Design review of the part built by this model. Coordinates are the model's own, in mm. Face numbers are marked on the shaded views. A direction names the side the tool comes from. Coordinates: 2 decimals unless noted, no trailing zeros. Order: outer loops, then holes, each group sorted by start corner. A loop starts at its lowest first (then second) coordinate and runs counter-clockwise, first axis right, second up. Notation, with made-up numbers: (32.5, -6) -> (86.5, -6) arc R19 cw to (86.5, 25) -> close; hole circle Ø1 at (13, -5). An arc over 180 degrees is marked (long way). Write item = value, one per line.
```python
from build123d import *

# Parameters (mm, degrees)
SCHIZZO1_W                        = 69
SCHIZZO1_H                        = 49
ESTRUSIONE_ESTRUSIONE1_DEPTH      = 3
RACCORDO1_R                       = 1
RACCORDO2_R                       = 1
RACCORDO3_R                       = 1
RACCORDO4_R                       = 1
SCHIZZO2_W                        = 60
SCHIZZO2_H                        = 2.231214474
ESTRUSIONE_ESTRUSIONE2_DEPTH      = 3
RACCORDO5_R                       = 3
RACCORDO6_R                       = 3
SCHIZZO3_R                        = 1
TAGLIO_ESTRUSIONE1_DEPTH          = 3
SCHIZZO4_W                        = 24
SCHIZZO4_H                        = 14
TAGLIO_ESTRUSIONE2_DEPTH          = 3
SCHIZZO5_W                        = 23
SCHIZZO5_H                        = 23
TAGLIO_ESTRUSIONE3_DEPTH          = 1.2
RACCORDO7_R                       = 0.5
RACCORDO8_R                       = 0.5
RACCORDO9_R                       = 0.5
RACCORDO10_R                      = 0.5
RACCORDO11_R                      = 2
RACCORDO12_R                      = 2
RACCORDO13_R                      = 2
RACCORDO14_R                      = 2
SCHIZZO6_W                        = 8.444052449
SCHIZZO6_H                        = 8.25
ESTRUSIONE_ESTRUSIONE3_DEPTH      = 6
SCHIZZO7_R                        = 0.9
TAGLIO_ESTRUSIONE4_DEPTH          = 6
ESTRUSIONE_ESTRUSIONE4_DEPTH      = 1.2
ESTRUSIONE_ESTRUSIONE4_DEPTH_BACK = 3
SCHIZZO8_R                        = 1.75
TAGLIO_ESTRUSIONE5_DEPTH          = 3
TAGLIO_ESTRUSIONE6_DEPTH          = 2
SCHIZZO13_R                       = 1.9
ESTRUSIONE_ESTRUSIONE5_DEPTH      = 3.2
SCHIZZO14_R                       = 1.9
ESTRUSIONE_ESTRUSIONE6_DEPTH      = 3.2


with BuildPart() as part:
    # Schizzo1 → Estrusione-Estrusione1 (new body)
    with BuildSketch(Plane(origin=(0, 0, 0), x_dir=(1, 0, 0), z_dir=(0, 1, 0))):
        Rectangle(SCHIZZO1_W, SCHIZZO1_H)
    extrude(amount=ESTRUSIONE_ESTRUSIONE1_DEPTH)

    # Raccordo1
    raccordo1_edges = [part.edges().sort_by_distance(p)[0] for p in [
        (-34.5, 1.5, 24.5),
    ]]
    fillet(raccordo1_edges, radius=RACCORDO1_R)

    # Raccordo2
    raccordo2_edges = [part.edges().sort_by_distance(p)[0] for p in [
        (-34.5, 1.5, -24.5),
    ]]
    fillet(raccordo2_edges, radius=RACCORDO2_R)

    # Raccordo3
    raccordo3_edges = [part.edges().sort_by_distance(p)[0] for p in [
        (34.5, 1.5, 24.5),
    ]]
    fillet(raccordo3_edges, radius=RACCORDO3_R)

    # Raccordo4
    raccordo4_edges = [part.edges().sort_by_distance(p)[0] for p in [
        (34.5, 1.5, -24.5),
    ]]
    fillet(raccordo4_edges, radius=RACCORDO4_R)

    # Schizzo2 → Estrusione-Estrusione2 (add)
    with BuildSketch(Plane.XZ):
        with Locations((0, 21.334392763)):
            Rectangle(SCHIZZO2_W, SCHIZZO2_H)
        with Locations((0, -21.334392763)):
            Rectangle(SCHIZZO2_W, SCHIZZO2_H)
    extrude(amount=ESTRUSIONE_ESTRUSIONE2_DEPTH)

    # Raccordo5
    raccordo5_edges = [part.edges().sort_by_distance(p)[0] for p in [
        (0, 0, 20.218785526),
    ]]
    fillet(raccordo5_edges, radius=RACCORDO5_R - 0.0001)  # a hair under: the kernel refuses the full size

    # Raccordo6
    raccordo6_edges = [part.edges().sort_by_distance(p)[0] for p in [
        (0, 0, -20.218785526),
    ]]
    fillet(raccordo6_edges, radius=RACCORDO6_R - 0.0001)  # a hair under: the kernel refuses the full size

    # Schizzo3 → Taglio-Estrusione1 (cut)
    with BuildSketch(Plane(origin=(0, 3, 0), x_dir=(1, 0, 0), z_dir=(0, 1, 0))):
        with Locations(Location((-32.5, 22.5, 0), (0, 0, 270))):
            Circle(SCHIZZO3_R)
        with Locations(Location((32.5, 22.5, 0), (0, 0, 270))):
            Circle(SCHIZZO3_R)
        with Locations(Location((32.5, -22.5, 0), (0, 0, 270))):
            Circle(SCHIZZO3_R)
        with Locations(Location((-32.5, -22.5, 0), (0, 0, 270))):
            Circle(SCHIZZO3_R)
    extrude(amount=-TAGLIO_ESTRUSIONE1_DEPTH, mode=Mode.SUBTRACT)

    # Schizzo4 → Taglio-Estrusione2 (cut)
    with BuildSketch(Plane.XZ):
        with Locations((9.5, 0)):
            Rectangle(SCHIZZO4_W, SCHIZZO4_H)
    extrude(amount=-TAGLIO_ESTRUSIONE2_DEPTH, mode=Mode.SUBTRACT)

    # Schizzo5 → Taglio-Estrusione3 (cut)
    with BuildSketch(Plane.XZ):
        with Locations((-21.5, 0)):
            Rectangle(SCHIZZO5_W, SCHIZZO5_H)
    extrude(amount=-TAGLIO_ESTRUSIONE3_DEPTH, mode=Mode.SUBTRACT)

    # Raccordo7
    raccordo7_edges = [part.edges().sort_by_distance(p)[0] for p in [
        (-33, 0.6, 11.5),
    ]]
    fillet(raccordo7_edges, radius=RACCORDO7_R)

    # Raccordo8
    raccordo8_edges = [part.edges().sort_by_distance(p)[0] for p in [
        (-10, 0.6, 11.5),
    ]]
    fillet(raccordo8_edges, radius=RACCORDO8_R)

    # Raccordo9
    raccordo9_edges = [part.edges().sort_by_distance(p)[0] for p in [
        (-33, 0.6, -11.5),
    ]]
    fillet(raccordo9_edges, radius=RACCORDO9_R)

    # Raccordo10
    raccordo10_edges = [part.edges().sort_by_distance(p)[0] for p in [
        (-10, 0.6, -11.5),
    ]]
    fillet(raccordo10_edges, radius=RACCORDO10_R)

    # Raccordo11
    raccordo11_edges = [part.edges().sort_by_distance(p)[0] for p in [
        (21.5, 3, 0),
    ]]
    fillet(raccordo11_edges, radius=RACCORDO11_R)

    # Raccordo12
    raccordo12_edges = [part.edges().sort_by_distance(p)[0] for p in [
        (10.5, 3, 7),
    ]]
    fillet(raccordo12_edges, radius=RACCORDO12_R)

    # Raccordo13
    raccordo13_edges = [part.edges().sort_by_distance(p)[0] for p in [
        (-2.5, 3, 1),
    ]]
    fillet(raccordo13_edges, radius=RACCORDO13_R)

    # Raccordo14
    raccordo14_edges = [part.edges().sort_by_distance(p)[0] for p in [
        (9.5, 3, -7),
    ]]
    fillet(raccordo14_edges, radius=RACCORDO14_R)

    # Schizzo6 → Estrusione-Estrusione3 (add)
    with BuildSketch(Plane.XZ):
        with Locations((-6.722026225, 18.375)):
            Rectangle(SCHIZZO6_W, SCHIZZO6_H)
        with Locations((-6.722026225, -18.375)):
            Rectangle(SCHIZZO6_W, SCHIZZO6_H)
    extrude(amount=ESTRUSIONE_ESTRUSIONE3_DEPTH)

    # Schizzo7 → Taglio-Estrusione4 (cut)
    with BuildSketch(Plane.XZ.offset(6)):
        with Locations(Location((-6.72, 18.375, 0), (0, 0, 270))):
            Circle(SCHIZZO7_R)
        with Locations(Location((-6.72, -18.375, 0), (0, 0, 90))):
            Circle(SCHIZZO7_R)
    extrude(amount=-TAGLIO_ESTRUSIONE4_DEPTH, mode=Mode.SUBTRACT)

    # Schizzo8 → Estrusione-Estrusione4 (add, two sides: drawn at the far end of the back side and taken through both)
    with BuildSketch(Plane.XZ.offset(-ESTRUSIONE_ESTRUSIONE4_DEPTH_BACK)):
        with Locations(Location((28.5, 8.7, 0), (0, 0, 270))):
            Circle(SCHIZZO8_R)
        with Locations(Location((28.5, -8.7, 0), (0, 0, 90))):
            Circle(SCHIZZO8_R)
    extrude(amount=ESTRUSIONE_ESTRUSIONE4_DEPTH + ESTRUSIONE_ESTRUSIONE4_DEPTH_BACK)

    # Schizzo9 → Taglio-Estrusione5 (cut)
    with BuildSketch(Plane.XZ):
        with BuildLine():
            Line((28.523054823, 11.139507375), (23.522221501, 11.139507375))
            Line((23.522221501, 11.139507375), (23.522221501, 11.920576973))
            Line((23.522221501, 11.920576973), (28.476945177, 11.920576973))
            ThreePointArc((28.476945177, 11.920576973), (30.793594038, 10.980088836), (31.766686618, 8.676945177))
            ThreePointArc((31.766686618, 8.676945177), (30.793594038, 6.373801519), (28.476945177, 5.433313382))
            Line((28.476945177, 5.433313382), (23.522221501, 5.433313382))
            Line((23.522221501, 5.433313382), (23.522221501, 6.21438298))
            Line((23.522221501, 6.21438298), (28.523054823, 6.21438298))
            ThreePointArc((28.523054823, 6.21438298), (30.241294429, 6.945200369), (30.939507375, 8.676945177))
            ThreePointArc((30.939507375, 8.676945177), (30.241294429, 10.408689986), (28.523054823, 11.139507375))
        make_face()
        with BuildLine():
            Line((23.522221501, -5.433313382), (23.522221501, -6.21438298))
            Line((23.522221501, -6.21438298), (28.523054823, -6.21438298))
            ThreePointArc((28.523054823, -6.21438298), (30.241294429, -6.945200369), (30.939507375, -8.676945177))
            ThreePointArc((30.939507375, -8.676945177), (30.241294429, -10.408689986), (28.523054823, -11.139507375))
            Line((28.523054823, -11.139507375), (23.522221501, -11.139507375))
            Line((23.522221501, -11.139507375), (23.522221501, -11.920576973))
            Line((23.522221501, -11.920576973), (28.476945177, -11.920576973))
            ThreePointArc((28.476945177, -11.920576973), (30.793594038, -10.980088836), (31.766686618, -8.676945177))
            ThreePointArc((31.766686618, -8.676945177), (30.793594038, -6.373801519), (28.476945177, -5.433313382))
            Line((28.476945177, -5.433313382), (23.522221501, -5.433313382))
        make_face()
    extrude(amount=-TAGLIO_ESTRUSIONE5_DEPTH, mode=Mode.SUBTRACT)

    # Schizzo11 → Taglio-Estrusione6 (cut)
    with BuildSketch(Plane.XZ):
        with BuildLine():
            Line((28.523054823, 11.139507375), (23.522221501, 11.139507375))
            Line((23.522221501, 11.139507375), (23.522221501, 6.21438298))
            Line((23.522221501, 6.21438298), (28.523054823, 6.21438298))
            ThreePointArc((28.523054823, 6.21438298), (30.248124061, 6.938498616), (30.939507375, 8.676945177))
            ThreePointArc((30.939507375, 8.676945177), (30.248124061, 10.415391738), (28.523054823, 11.139507375))
        make_face()
        with BuildLine():
            Line((23.522221501, -6.21438298), (28.523054823, -6.21438298))
            ThreePointArc((28.523054823, -6.21438298), (30.248124061, -6.938498616), (30.939507375, -8.676945177))
            ThreePointArc((30.939507375, -8.676945177), (30.248124061, -10.415391738), (28.523054823, -11.139507375))
            Line((28.523054823, -11.139507375), (23.522221501, -11.139507375))
            Line((23.522221501, -11.139507375), (23.522221501, -6.21438298))
        make_face()
    extrude(amount=-TAGLIO_ESTRUSIONE6_DEPTH, mode=Mode.SUBTRACT)


with BuildPart() as taglio_estrusione6_piece_1:
    # of the separate pieces the step leaves, piece 1, a body of its own (taglio_estrusione6_pieces)
    add(part.part.solids().sort_by_distance((34.5, 3, -23.5))[0])



with BuildPart() as taglio_estrusione6_piece_2:
    # of the separate pieces the step leaves, piece 2, a body of its own (taglio_estrusione6_pieces)
    add(part.part.solids().sort_by_distance((28.5, 0, 6.95))[0])


with BuildPart() as taglio_estrusione6_piece_3:
    # of the separate pieces the step leaves, piece 3, a body of its own (taglio_estrusione6_pieces)
    add(part.part.solids().sort_by_distance((28.5, 0, -6.95))[0])


with BuildPart() as taglio_estrusione6_piece_1_1:
    add(taglio_estrusione6_piece_1.part)

    add(taglio_estrusione6_piece_2.part)  # Estrusione-Estrusione5 merges Taglio-Estrusione6 piece 2
    # Schizzo13 → Estrusione-Estrusione5 (add)
    with BuildSketch(Plane.XZ.offset(-2)):
        with Locations(Location((28.5, 8.7, 0), (0, 0, 90))):
            Circle(SCHIZZO13_R)
    extrude(amount=ESTRUSIONE_ESTRUSIONE5_DEPTH)


    add(taglio_estrusione6_piece_3.part)  # Estrusione-Estrusione6 merges Taglio-Estrusione6 piece 3
    # Schizzo14 → Estrusione-Estrusione6 (add)
    with BuildSketch(Plane.XZ.offset(-2)):
        with Locations(Location((28.5, -8.7, 0), (0, 0, 90))):
            Circle(SCHIZZO14_R)
    extrude(amount=ESTRUSIONE_ESTRUSIONE6_DEPTH)


solid = taglio_estrusione6_piece_1_1.part
```
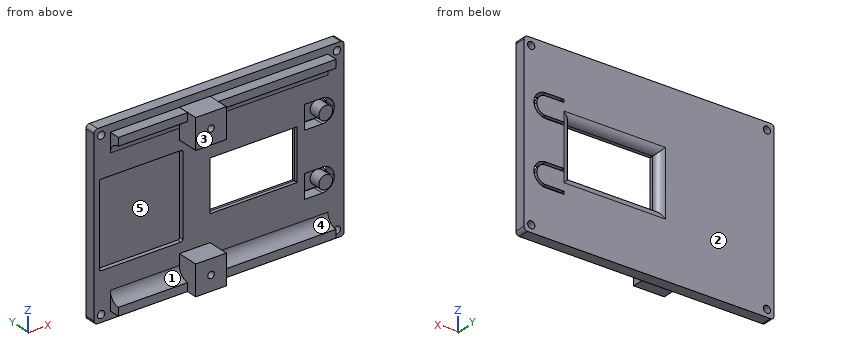
(1) For the marked faces 3, 4 and 5, list the 3-axis set-ups (+Z, -Z, +X, -X, +Y, -Y) from which the entire face can be reached by the end or side of a thin tool; tool diameter is ignored.
Report:
face_3 = +Z, -Z, +X, -X, -Y
face_4 = +X, -Y
face_5 = -Y
(2) We need section A-A (x = 32.5). Write out the cut boundary in (y, z).
Report:
outline = (0, -24.5) -> (3, -24.5) -> (3, -23.5) -> (0, -23.5) -> close; (0, -21.5) -> (3, -21.5) -> (3, 21.5) -> (0, 21.5) -> close; (0, 23.5) -> (3, 23.5) -> (3, 24.5) -> (0, 24.5) -> close
(3) For L1, parallel to X at y = 1.75, z = -22.5; L2, parallel to Z at x = -9, y = -3; L3, parallel to Z at x = 29, y = 1.5, list the stretches that pass through material, from the lowest coordinate up.
Report:
L1 = -34.5 to -33.5, -31.5 to 31.5, 33.5 to 34.5
L2 = -22.5 to -14.25, 14.25 to 22.5
L3 = -24.5 to -11.88, -10.53 to -6.87, -5.47 to 5.47, 6.87 to 10.53, 11.88 to 24.5
(4) The part is to be moulded in two halves that separate along Z. For the marked faces 1 and 2, say which applies: released by +Z, released by -Z, zero draft, split by the parting line, or undercut.
Report:
face_1 = undercut
face_2 = zero draft
(5) We need section D-D (x = -6.72). Write out the cut boundary in (y, z) (3 decimals).
Report:
outline = (-6, -22.5) -> (0, -22.5) -> (0, -24.5) -> (3, -24.5) -> (3, 24.5) -> (0, 24.5) -> (0, 22.5) -> (-6, 22.5) -> (-6, 19.275) -> (0, 19.275) -> (0, 17.475) -> (-6, 17.475) -> (-6, 14.25) -> (0, 14.25) -> (0, -14.25) -> (-6, -14.25) -> (-6, -17.475) -> (0, -17.475) -> (0, -19.275) -> (-6, -19.275) -> close
(6) We need section B-B (z = -2.5). Write out the cut boundary in (x, y), and give its area (3 significant figures).
Report:
outline = (-34.5, 0) -> (-33, 0) -> (-33, 1.2) -> (-10, 1.2) -> (-10, 0) -> (-2.5, 0) -> (-2.5, 1) arc R2 ccw to (-4.5, 3) -> (-34.5, 3) -> close; (21.5, 0) -> (34.5, 0) -> (34.5, 3) -> (23.5, 3) arc R2 ccw to (21.5, 1) -> close
area = 106 mm²
(7) Insertion check: pin 1 (1.5 mm diameter, centred on y = -2, z = 19, fed in from -X); pin 2 (24.5 mm diameter, centred on x = -9.5, z = -8.5, fed in from -Y); pin 3 (0.7 mm diameter, centred on x = -17.5, z = -21, fed in from -Y); pin 4 (6 mm diameter, centred on x = 27.5, z = -2.5, fed in from -Y). Each pin has a flat end and moves straight along its axis. Give the tip position at first contact, or say it passes through.
Report:
pin_1 = -10.94
pin_2 = -6
pin_3 = -3
pin_4 = 0
(8) We need section C-C (x = 24.5). Give the number of separate pieces and of enclosed holes in the cut face, and give its area (3 significant figures).
Report:
separate_pieces = 5
enclosed_holes = 0
area = 135 mm²
